Could you check a few things on this drawing? It's one solid part, dimensions in mm from its lowest x, y, z. A direction names the side the tool comes from. Give positions to 0.01 mm unless a question says otherwise; leave off trailing zeros. Order: outer loops, then holes, each group sorted by start corner. A loop starts at its lowest first (then second) coordinate and runs counter-clockwise, first axis right, second up. Notation, with made-up numbers: M -26.75,-22 L 0.25,-22 A30 cw 0.25,9 Z; hole C 84.25,82.25 d9. An arc over 180 degrees is marked long. One line per item, written item: value. Start each with the question number.
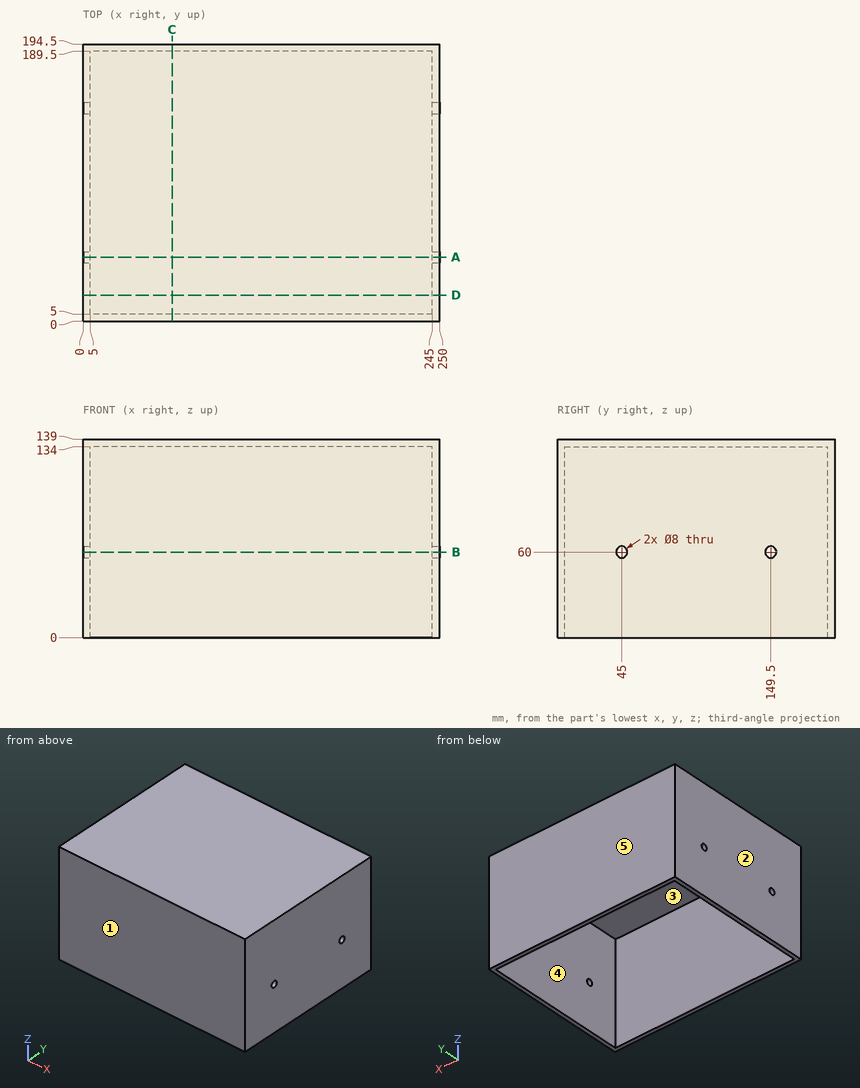
Item 1: I want a section at D-D on y = 18.5. Write out the boundary of the cut face in (x, z).
Item 2: I want a section at C-C on x = 62.5. Write out the boundary of the cut face in (y, z).
Item 3: Will these pins go through, and if not, where does the flat tip stop? P1, Ø5, axis at y = 45, z = 60, coming from the +X side; P2, Ø1.5, axis at x = 27, y = 43.5, coming from the -Z side.
Item 4: For the marked faces 4 and 5, which set-ups out of +Z, -Z, +X, -X, +Y, -Y let a thin tool reach every point of the face, with its end or its side?
Item 5: I want a section at B-B on z = 60. Write out the boundary of the cut face in (x, y), plus the area to 4 significant figures.
Item 6: Please list where these lines run through material, in increasing order: probe 1 along Y at (x, z) = (246.35, 60); probe 2 along X at (y, z) = (139, 114); probe 3 along Y at (x, z) = (174, 81.5). Write a range as [from, to].
Item 7: I want a section at A-A on y = 45. Write out the boundary of the cut face in (x, z).
Item 8: We'd pull the mould along X, two halves only. Please class the marked faces 1, 2 and 3: +X half, -X half, draft (parallel to the pull), parting line (faces both ways), or undercut.
Answer below:
1. outline: M 0,0 L 5,0 L 5,134 L 245,134 L 245,0 L 250,0 L 250,139 L 0,139 Z
2. outline: M 0,0 L 5,0 L 5,134 L 189.5,134 L 189.5,0 L 194.5,0 L 194.5,139 L 0,139 Z
3. P1: passes through
3. P2: stops at z = 134
4. face 4: -Z
4. face 5: +Z, -Z, +X, -X, +Y
5. outline: M 0,0 L 250,0 L 250,41 L 245,41 L 245,5 L 5,5 L 5,41 L 0,41 Z; M 0,49 L 5,49 L 5,145.5 L 0,145.5 Z; M 0,153.5 L 5,153.5 L 5,189.5 L 245,189.5 L 245,153.5 L 250,153.5 L 250,194.5 L 0,194.5 Z; M 245,49 L 250,49 L 250,145.5 L 245,145.5 Z
5. area: 4,185 mm²
6. probe 1: y = [0, 41], [49, 145.5], [153.5, 194.5]
6. probe 2: x = [0, 5], [245, 250]
6. probe 3: y = [0, 5], [189.5, 194.5]
7. outline: M 0,0 L 5,0 L 5,56 L 0,56 Z; M 0,64 L 5,64 L 5,134 L 245,134 L 245,64 L 250,64 L 250,139 L 0,139 Z; M 245,0 L 250,0 L 250,56 L 245,56 Z
8. face 1: draft
8. face 2: -X half
8. face 3: undercut
